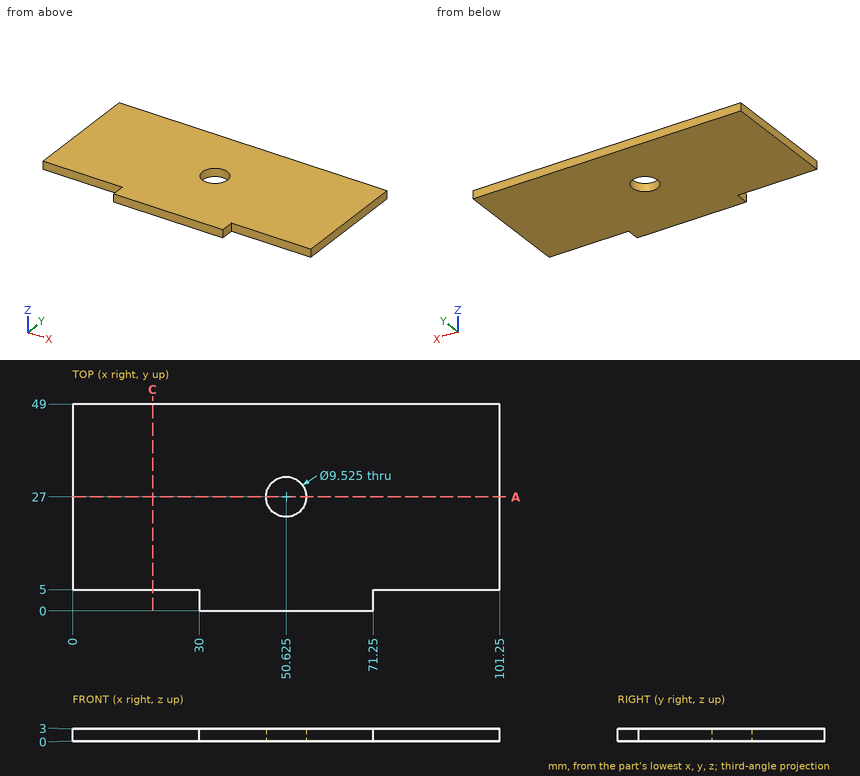
Part print with two shaded views. Sizes in mm from the minimum x, y, z corner. Coordinates: 2 decimals unless noted, no trailing zeros. Order: outer loops, then holes, each group sorted by start corner. A loop starts at its lowest first (then second) coordinate and runs counter-clockwise, first axis right, second up. Notation, with made-up numbers: (-9, 8.25) - (36, 8.25) arc R22 cw to (36, 41.25) - close; hole circle Ø10 at (-34.75, 33.5). An arc over 180 degrees is marked (long way). Write item = value, one per line. Start each with the question number.
1) Saw through at C-C on x = 19. Write the cut outline in (y, z), then the cut area to 3 significant figures.
2) Wall check: line 1 along X through (y, z) = (4, 1.3); line 2 along Y through (x, z) = (22.5, 0.6); line 3 along X through (y, z) = (29, 0.25). Give the ranges that are in metal, low to high. Write a range as from..to.
3) Flat gauge pins, fed straight in: pin 1 Ø1.5 at (x, z) = (21, 1) entering from -Y; pin 2 Ø0.9 at (y, z) = (2.5, 1) entering from +X; pin 3 Ø1.5 at (y, z) = (1.5, 1.5) entering from -X. Where does each tip first touch, or does it go through?
4) Saw through at A-A on y = 27. Write the cut outline in (x, z).
From the geometry:
q1.outline = (5, 0) - (49, 0) - (49, 3) - (5, 3) - close
q1.area = 132 mm^2
q2.line_1 = 30..71.25
q2.line_2 = 5..49
q2.line_3 = 0..46.3, 54.95..101.25
q3.pin_1 = 5
q3.pin_2 = 71.25
q3.pin_3 = 30
q4.outline = (0, 0) - (45.86, 0) - (45.86, 3) - (0, 3) - close; (55.39, 0) - (101.25, 0) - (101.25, 3) - (55.39, 3) - close
